Design review of the part built by this model. Coordinates are the model's own, in mm. Face numbers are marked on the shaded views. A direction names the side the tool comes from. Give positions to 0.01 mm unless a question says otherwise; leave off trailing zeros. Write each loop counter-clockwise with the first axis right and the second up, starting at its lowest first coordinate (ties: lowest second). Pieces come first, ordered by that corner, then holes. Notation, with made-up numbers: M -20,-35.75 L 11,-35.75 A16 ccw 11,-14.75 Z; hole C 27.25,53.5 d4. An arc over 180 degrees is marked long. Use a Markdown table: item, result. Add a question column.
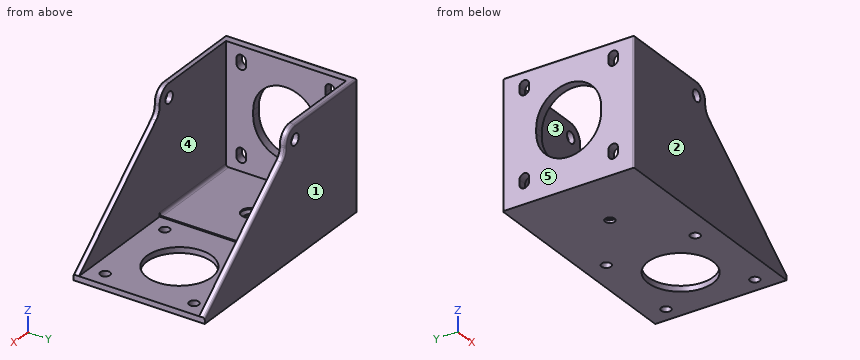
```python
from build123d import *

# Parameters (mm, degrees)
SKETCH_1_W               = 42.6
SKETCH_1_H               = 42.6
SKETCH_1_R               = 1.7
SKETCH_1_R_2             = 11.5
EXTRUDE_1_DEPTH          = 2
SKETCH_2_W               = 37
SKETCH_2_H               = 42.6
EXTRUDE_2_DEPTH          = 2
EXTRUDE_3_DEPTH          = 2
EXTRUDE_4_DEPTH          = 2
BOSS_EXTRUDE1_DEPTH      = 36
BOSS_EXTRUDE1_DEPTH_BACK = 2
SKETCH1_W                = 44.957073211
SKETCH1_H                = 46.6
SKETCH4_W                = 35
SKETCH4_H                = 42.6
CUT_EXTRUDE2_DEPTH       = 42.5
CUT_EXTRUDE3_REACH       = 97.186
CUT_EXTRUDE4_REACH       = 79.978
SKETCH6_R                = 1.7
SKETCH7_R                = 3
CUT_EXTRUDE5_DEPTH       = 1.5
FILLET1_R                = 5
FILLET2_R                = 1
CHAMFER1_SIZE            = 1
FILLET3_R                = 0.6
SKETCH8_R                = 2
CUT_EXTRUDE6_DEPTH       = 88.801984213


with BuildPart() as part:
    # Эскиз1 → Бобышка-Вытянуть1 (new body)
    with BuildSketch(Plane.XY):
        Rectangle(SKETCH_1_W, SKETCH_1_H)
        with Locations((-15.75, 15.75)):
            Circle(SKETCH_1_R, mode=Mode.SUBTRACT)
        with Locations((15.75, 15.75)):
            Circle(SKETCH_1_R, mode=Mode.SUBTRACT)
        with Locations((15.75, -15.75)):
            Circle(SKETCH_1_R, mode=Mode.SUBTRACT)
        with Locations((-15.75, -15.75)):
            Circle(SKETCH_1_R, mode=Mode.SUBTRACT)
        Circle(SKETCH_1_R_2, mode=Mode.SUBTRACT)
    extrude(amount=EXTRUDE_1_DEPTH)

    # Эскиз2 → Бобышка-Вытянуть2 (add)
    with BuildSketch(Plane.ZY.offset(21.3)):
        with Locations((18.5, 0)):
            Rectangle(SKETCH_2_W, SKETCH_2_H)
    extrude(amount=EXTRUDE_2_DEPTH)

    # Эскиз3 → Бобышка-Вытянуть3 (add)
    with BuildSketch(Plane.XZ.offset(21.3)):
        Polygon((-23.3, 0), (-23.3, 37), (-21.3, 37), (21.3, 2), (21.3, 0), align=None)
    extrude(amount=EXTRUDE_3_DEPTH)

    # Эскиз4 → Бобышка-Вытянуть4 (add)
    with BuildSketch(Plane(origin=(0, 21.3, 0), x_dir=(1, 0, 0), z_dir=(0, 1, 0))):
        Polygon((-23.3, -37), (-23.3, 0), (21.3, 0), (21.3, -2), (-21.3, -37), align=None)
    extrude(amount=EXTRUDE_4_DEPTH)

    # Sketch1 → Boss-Extrude1 (add, two sides: drawn at the far end of the back side and taken through both)
    with BuildSketch(Plane.ZY.offset(23.3).offset(-BOSS_EXTRUDE1_DEPTH_BACK)):
        with Locations((22.478536606, 0)):
            Rectangle(SKETCH1_W, SKETCH1_H)
    extrude(amount=BOSS_EXTRUDE1_DEPTH + BOSS_EXTRUDE1_DEPTH_BACK)

    # Sketch4 → Cut-Extrude2 (cut)
    with BuildSketch(Plane.XY.offset(44.957073211)):
        with Locations((-38.8, 0)):
            Rectangle(SKETCH4_W, SKETCH4_H)
    extrude(amount=-CUT_EXTRUDE2_DEPTH, mode=Mode.SUBTRACT)

    # Sketch5 → Cut-Extrude3 (cut, up to next)
    with BuildSketch(Plane.ZY.offset(59.3), mode=Mode.PRIVATE) as cut_extrude3_sk1:
        with BuildLine():
            Line((38.570845355, -14.202343453), (40.270845355, -14.202343453))
            ThreePointArc((40.270845355, -14.202343453), (41.970845355, -15.902343453), (40.270845355, -17.602343453))
            Line((40.270845355, -17.602343453), (38.570845355, -17.602343453))
            ThreePointArc((38.570845355, -17.602343453), (36.870845355, -15.902343453), (38.570845355, -14.202343453))
        make_face()
    cut_extrude3_tool1 = extrude(cut_extrude3_sk1.sketch, amount=-CUT_EXTRUDE3_REACH, mode=Mode.PRIVATE) & part.part
    # Sketch5 → Cut-Extrude3 (cut, up to next)
    with BuildSketch(Plane.ZY.offset(59.3), mode=Mode.PRIVATE) as cut_extrude3_sk2:
        with BuildLine():
            Line((38.570845355, 13.897656547), (40.270845355, 13.897656547))
            ThreePointArc((40.270845355, 13.897656547), (41.970845355, 15.597656547), (40.270845355, 17.297656547))
            Line((40.270845355, 17.297656547), (38.570845355, 17.297656547))
            ThreePointArc((38.570845355, 17.297656547), (36.870845355, 15.597656547), (38.570845355, 13.897656547))
        make_face()
    cut_extrude3_tool2 = extrude(cut_extrude3_sk2.sketch, amount=-CUT_EXTRUDE3_REACH, mode=Mode.PRIVATE) & part.part
    # Sketch5 → Cut-Extrude3 (cut, up to next)
    with BuildSketch(Plane.ZY.offset(59.3), mode=Mode.PRIVATE) as cut_extrude3_sk3:
        with BuildLine():
            Line((7.070845355, 17.297656547), (8.770845355, 17.297656547))
            ThreePointArc((8.770845355, 17.297656547), (10.470845355, 15.597656547), (8.770845355, 13.897656547))
            Line((8.770845355, 13.897656547), (7.070845355, 13.897656547))
            ThreePointArc((7.070845355, 13.897656547), (5.370845355, 15.597656547), (7.070845355, 17.297656547))
        make_face()
    cut_extrude3_tool3 = extrude(cut_extrude3_sk3.sketch, amount=-CUT_EXTRUDE3_REACH, mode=Mode.PRIVATE) & part.part
    # Sketch5 → Cut-Extrude3 (cut, up to next)
    with BuildSketch(Plane.ZY.offset(59.3), mode=Mode.PRIVATE) as cut_extrude3_sk4:
        with BuildLine():
            Line((7.070845355, -14.202343453), (8.770845355, -14.202343453))
            ThreePointArc((8.770845355, -14.202343453), (10.470845355, -15.902343453), (8.770845355, -17.602343453))
            Line((8.770845355, -17.602343453), (7.070845355, -17.602343453))
            ThreePointArc((7.070845355, -17.602343453), (5.370845355, -15.902343453), (7.070845355, -14.202343453))
        make_face()
    cut_extrude3_tool4 = extrude(cut_extrude3_sk4.sketch, amount=-CUT_EXTRUDE3_REACH, mode=Mode.PRIVATE) & part.part
    # Sketch5 → Cut-Extrude3 (cut, up to next)
    with BuildSketch(Plane.ZY.offset(59.3), mode=Mode.PRIVATE) as cut_extrude3_sk5:
        with BuildLine():
            Line((22.520845355, 11.347656547), (24.520845355, 11.347656547))
            ThreePointArc((24.520845355, 11.347656547), (36.020845355, -0.152343453), (24.520845355, -11.652343453))
            Line((24.520845355, -11.652343453), (22.520845355, -11.652343453))
            ThreePointArc((22.520845355, -11.652343453), (11.020845355, -0.152343453), (22.520845355, 11.347656547))
        make_face()
    cut_extrude3_tool5 = extrude(cut_extrude3_sk5.sketch, amount=-CUT_EXTRUDE3_REACH, mode=Mode.PRIVATE) & part.part
    add(cut_extrude3_tool1.solids().sort_by_distance((-59.3, -15.902343, 39.420845))[0], mode=Mode.SUBTRACT)
    add(cut_extrude3_tool2.solids().sort_by_distance((-59.3, 15.597657, 39.420845))[0], mode=Mode.SUBTRACT)
    add(cut_extrude3_tool3.solids().sort_by_distance((-59.3, 15.597657, 7.920845))[0], mode=Mode.SUBTRACT)
    add(cut_extrude3_tool4.solids().sort_by_distance((-59.3, -15.902343, 7.920845))[0], mode=Mode.SUBTRACT)
    add(cut_extrude3_tool5.solids().sort_by_distance((-59.3, -0.152343, 23.520845))[0], mode=Mode.SUBTRACT)

    # Sketch6 → Cut-Extrude4 (cut, up to next)
    with BuildSketch(Plane(origin=(0, 0, 0), x_dir=(-1, 0, 0), z_dir=(0, 0, -1)), mode=Mode.PRIVATE) as cut_extrude4_sk1:
        with Locations((37.3, 0)):
            Circle(SKETCH6_R)
    cut_extrude4_tool1 = extrude(cut_extrude4_sk1.sketch, amount=-CUT_EXTRUDE4_REACH, mode=Mode.PRIVATE) & part.part
    add(cut_extrude4_tool1.solids().sort_by_distance((-37.3, 0, 0))[0], mode=Mode.SUBTRACT)

    # Sketch7 → Cut-Extrude5 (cut)
    with BuildSketch(Plane.XY.offset(2.457073211)):
        with Locations((-37.3, 0)):
            Circle(SKETCH7_R)
    extrude(amount=-CUT_EXTRUDE5_DEPTH, mode=Mode.SUBTRACT)

    # Fillet1
    fillet1_edges = [part.edges().sort_by_distance(p)[0] for p in [
        (-21.3, 22.3, 44.957073211),
        (-21.3, -22.3, 37),
        (-21.3, 22.3, 37),
        (-21.3, -22.3, 44.957073211),
    ]]
    fillet(fillet1_edges, radius=FILLET1_R)

    # Fillet2
    fillet2_edges = [part.edges().sort_by_distance(p)[0] for p in [
        (-38.8, -21.3, 2.457073211),
        (-38.8, 21.3, 2.457073211),
    ]]
    fillet(fillet2_edges, radius=FILLET2_R)

    # Chamfer1
    chamfer1_edges = [part.edges().sort_by_distance(p)[0] for p in [
        (-40.3, 0, 0.957073211),
    ]]
    chamfer(chamfer1_edges, length=CHAMFER1_SIZE)

    # Fillet3
    fillet3_edges = [part.edges().sort_by_distance(p)[0] for p in [
        (0.912958055, 23.3, 18.749917091),
        (-21.3, 23.3, 39.660110463),
        (-21.3, -23.3, 39.660110463),
        (-42.8, 23.3, 44.957073211),
        (-42.8, -23.3, 44.957073211),
        (-22.764466094, -23.3, 43.492607117),
        (-22.764466094, 23.3, 43.492607117),
        (-20.820532018, 23.3, 37.226610733),
        (-20.820532018, -23.3, 37.226610733),
        (0.912958055, -23.3, 18.749917091),
        (-59.3, -23.3, 22.478536605),
        (-59.3, 0, 44.957073211),
        (-59.3, 23.3, 22.478536605),
    ]]
    fillet(fillet3_edges, radius=FILLET3_R)

    # Sketch8 → Cut-Extrude6 (cut, through all)
    with BuildSketch(Plane.XZ.offset(23.3)):
        with Locations(Location((-26.3, 39.957073211, 0), (0, 0, 270))):
            Circle(SKETCH8_R)
    extrude(amount=-CUT_EXTRUDE6_DEPTH, mode=Mode.SUBTRACT)


solid = part.part
```
(1) For pin 1 (2 mm diameter, centred on x = -40, y = -18, fed in from +Z); pin 2 (2 mm diameter, centred on x = 15.75, y = 15.75, fed in from +Z); pin 3 (2 mm diameter, centred on y = 15, z = 14, fed in from +X); pin 4 (3 mm diameter, centred on x = -37, y = -0.5, fed in from +Z), all flat-tipped, find the tip position at first contact; note any pin that passes through.
(2) Add section A-A on y = 0. Give the boundary of the cut face in (x, z), then the cut area to 3 significant figures.
(3) Wall thickness on L1, parallel to Y at x = 15.75, z = 0.85; L2, parallel to Y at x = -52, z = 7; L3, parallel to Y at x = -37.3, z = 0.25: over which ranges is each line inside the solid? List them lowest first.
(4) Add section C-C on x = 15.75. Give the number of separate pieces and of enclosed holes in the cut face, then the cut area to 3 significant figures.
(5) The part is to be moulded in two halves that separate along Y. For the marked faces 1, 2 and 3, say which applies: released by +Y, released by -Y, zero draft, split by the parting line, or undercut.
(6) Machinability: for the marked faces 4 and 5, which of the approach directions +Z, -Z, +X, -X, +Y, -Y give a long, thin tool a straight path to every point of the face, cutting with its end or side? Answer none if there is none.
(7) Add section B-B on y = 15.75. Give the boundary of the cut face in (x, z).
From the geometry:
| question | item | result |
|---|---|---|
| 1 | pin 1 | stops at z = 2.46 |
| 1 | pin 2 | passes through |
| 1 | pin 3 | stops at x = -56.3 |
| 1 | pin 4 | stops at z = 1.04 |
| 2 | outline | M -59.3,0 L -39,0 L -39,0.96 L -39.3,0.96 L -40.3,1.96 L -40.3,2.46 L -56.3,2.46 L -56.3,11.02 L -59.3,11.02 Z; M -59.3,36.02 L -56.3,36.02 L -56.3,44.96 L -58.7,44.96 A0.6 ccw -59.3,44.36 Z; M -35.6,0 L -11.5,0 L -11.5,2 L -21.3,2 L -21.3,2.46 L -34.3,2.46 L -34.3,1.96 L -35.3,0.96 L -35.6,0.96 Z; M 11.5,0 L 21.3,0 L 21.3,2 L 11.5,2 Z |
| 2 | area | 174 mm^2 |
| 3 | L1 | y = -23.3 to -17.45, -14.05 to 14.05, 17.45 to 23.3 |
| 3 | L2 | y = -23.3 to -21.3, 21.3 to 23.3 |
| 3 | L3 | y = -23.3 to -1.7, 1.7 to 23.3 |
| 4 | separate pieces | 3 |
| 4 | enclosed holes | 0 |
| 4 | area | 97.6 mm^2 |
| 5 | face 1 | released by +Y |
| 5 | face 2 | released by -Y |
| 5 | face 3 | undercut |
| 6 | face 4 | +Z, +X |
| 6 | face 5 | +Z, -Z, -X, +Y, -Y |
| 7 | outline | M -59.3,0 L -17.45,0 L -17.45,2 L -21.3,2 L -21.3,2.46 L -56.3,2.46 L -56.3,5.38 L -59.3,5.38 Z; M -59.3,10.46 L -56.3,10.46 L -56.3,36.88 L -59.3,36.88 Z; M -59.3,41.96 L -56.3,41.96 L -56.3,44.96 L -58.7,44.96 A0.6 ccw -59.3,44.36 Z; M -14.05,0 L 14.05,0 L 14.05,2 L -14.05,2 Z; M 17.45,0 L 21.3,0 L 21.3,2 L 17.45,2 Z |
